```python
from build123d import *

# Parameters (mm, degrees)
F0_W     = 127
F0_H     = 50.8
F0_R     = 12.7
F1_DEPTH = 12.7
F2_W     = 6.35
F2_H     = 50.8
F3_DEPTH = 2.54
F5_DEPTH = 50.801
F6_R     = 4.7625
F7_DEPTH = 12.7


with BuildPart() as f1:
    # F0 (on Top) → F1 (new body)
    with BuildSketch(Plane.XY):
        Rectangle(F0_W, F0_H)
        Circle(F0_R, mode=Mode.SUBTRACT)
    extrude(amount=F1_DEPTH)

    # F2 (on face) → F3 (cut)
    with BuildSketch(Plane.XY.offset(12.7)):
        with BuildLine():
            Line((5.0018308049, 25.4), (-5.1581691951, 25.4))
            Line((-5.1581691951, 25.4), (-5.1581691951, 11.6053130313))
            ThreePointArc((-5.1581691951, 11.6053130313), (-0.0852899505, 12.699713604), (5.0018308049, 11.6735465305))
            Line((5.0018308049, 11.6735465305), (5.0018308049, 25.4))
        make_face()
        with BuildLine():
            Line((-5.1581691951, -11.6053130313), (-5.1581691951, -25.4))
            Line((-5.1581691951, -25.4), (5.0018308049, -25.4))
            Line((5.0018308049, -25.4), (5.0018308049, -11.6735465305))
            ThreePointArc((5.0018308049, -11.6735465305), (-0.0852899505, -12.699713604), (-5.1581691951, -11.6053130313))
        make_face()
        with Locations((-57.785, 0)):
            Rectangle(F2_W, F2_H)
    extrude(amount=-F3_DEPTH, mode=Mode.SUBTRACT)

    # F4 (on face) → F5 (cut, through all)
    with BuildSketch(Plane.XZ.offset(25.4)):
        Polygon((42.0720207126, 12.7), (29.3720207126, 12.7), (25.7058465033, 6.35), (45.738194922, 6.35), align=None)
    extrude(amount=-F5_DEPTH, mode=Mode.SUBTRACT)

    # F6 (on face) → F7 (join)
    with BuildSketch(Plane.YZ.offset(63.5)):
        with Locations((0, 6.35)):
            Circle(F6_R)
    extrude(amount=F7_DEPTH)


solid = f1.part
```
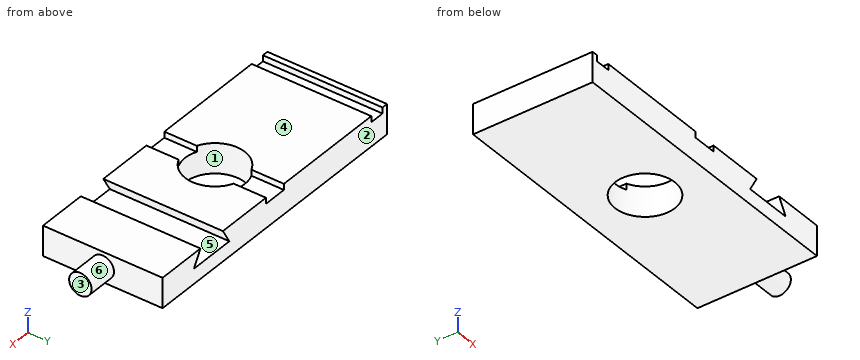
Geometry check sheet. Reference: the model listing, model coordinates, mm. Face numbers are marked on the shaded views. A direction names the side the tool comes from. Coordinates: 2 decimals unless noted, no trailing zeros. Order: outer loops, then holes, each group sorted by start corner. A loop starts at its lowest first (then second) coordinate and runs counter-clockwise, first axis right, second up. Notation, with made-up numbers: M 16,64.25 L 71,64.25 A37 cw 71,101.25 Z; hole C 46,-28 d11. An arc over 180 degrees is marked long. One line per question, with ' | ' between items. Start each with the question number.
Item 1: Material ranges on L1, parallel to X at y = -7, z = 11; L2, parallel to X at y = 0, z = 4.5; L3, parallel to Y at x = 0, z = 8.25, recorded low to high. Write a range as [from, to].
Item 2: Gauge pin test, flat ends, axial feed: pin 1 (1.3 mm diameter, centred on y = 21.5, z = 11.5, fed in from +X); pin 2 (1.9 mm diameter, centred on x = -59, y = 4, fed in from +Z); pin 3 (20.5 mm diameter, centred on x = 0, y = 0, fed in from +Z). Record the tip position at first contact, or that the pin passes through.
Item 3: Draft check along Y on the marked faces 1, 2 and 3. Enter one of: pulls with the +Y half, pulls with the -Y half, needs draft (parallel to the pull), parting line crosses it, or undercut.
Item 4: Cross-section at C-C on z = 4. Enter the section's corners in (x, y).
Item 5: Cross-section at D-D on y = -21.5. Enter the section's corners in (x, z), then the cut area to 3 significant figures.
Item 6: Cross-section at A-A on y = 0. Enter the section's corners in (x, z), then the cut area to 3 significant figures.
Item 7: Cross-section at B-B on x = 0. Enter the section's corners in (y, z).
Item 8: Set-up check for the marked faces 4, 5 and 6: record each of +Z, -Z, +X, -X, +Y, -Y from which the full face is reachable in a straight line by a thin tool's end or side.
Findings:
1) L1: x = [-63.5, -60.96], [-54.61, -10.6], [10.6, 28.39], [43.05, 63.5] | L2: x = [-63.5, -12.7], [12.7, 76.2] | L3: y = [-25.4, -12.7], [12.7, 25.4]
2) pin 1: stops at x = 63.5 | pin 2: stops at z = 10.16 | pin 3: passes through
3) face 1: undercut | face 2: pulls with the +Y half | face 3: needs draft
4) outline: M -63.5,-25.4 L 63.5,-25.4 L 63.5,-4.14 L 76.2,-4.14 L 76.2,4.14 L 63.5,4.14 L 63.5,25.4 L -63.5,25.4 Z; hole C 0,0 d25.4
5) outline: M -63.5,0 L 63.5,0 L 63.5,12.7 L 42.07,12.7 L 45.74,6.35 L 25.71,6.35 L 29.37,12.7 L 5,12.7 L 5,10.16 L -5.16,10.16 L -5.16,12.7 L -54.61,12.7 L -54.61,10.16 L -60.96,10.16 L -60.96,12.7 L -63.5,12.7 Z | area: 1,470 mm²
6) outline: M -63.5,0 L -12.7,0 L -12.7,12.7 L -54.61,12.7 L -54.61,10.16 L -60.96,10.16 L -60.96,12.7 L -63.5,12.7 Z; M 12.7,0 L 63.5,0 L 63.5,1.59 L 76.2,1.59 L 76.2,11.11 L 63.5,11.11 L 63.5,12.7 L 42.07,12.7 L 45.74,6.35 L 25.71,6.35 L 29.37,12.7 L 12.7,12.7 Z | area: 1,290 mm²
7) outline: M -25.4,0 L -12.7,0 L -12.7,10.16 L -25.4,10.16 Z; M 12.7,0 L 25.4,0 L 25.4,10.16 L 12.7,10.16 Z
8) face 4: +Z, +X, -X, +Y, -Y | face 5: +Y, -Y | face 6: +X
